Model file for the job. Use its own axes, mm. Round coordinates to 2 decimals unless told otherwise and drop trailing zeros. Loops run counter-clockwise (first coordinate to the right, second up) from the corner with the lowest first, then second, coordinate; pieces in that order, holes last. Notation, with made-up numbers: M 24.25,72 L 30.25,72 A8 ccw 30.25,82 Z; hole C 39.25,-1 d3. An arc over 180 degrees is marked long. Use a Markdown table: item, result. Add a question column.
Q1. Probe line 1 (X direction, y = -2, z = 36.5); line 2 (X direction, y = -4, z = 285). List the from-to ranges inside material, lowest first. Write a range as from..to.
Q2. Cut at B-B (x = 269.5). Give the cut face in (y, z), plus the area to 3 significant figures.
Q3. Cut at D-D (z = -49.5). Give the cut face in (x, y), plus the area to 3 significant figures.
Q4. Cut at A-A (z = 275). Give the cut face in (x, y).
Q5. Cut at C-C (y = -2.75). Give the cut face in (x, z), plus the area to 3 significant figures.
Q6. Pin check, flat tips, straight feed: pin 1 (1 mm diameter, centred on x = -131, y = -2, fed in from +Z); pin 2 (3 mm diameter, centred on x = 133.5, y = -1, fed in from -Z); pin 3 (1.5 mm diameter, centred on y = -2, z = 50.5, fed in from +X). Stop position of each tip, or through.
from build123d import *

# Parameters (mm, degrees)
BOSS_EXTRUDE1_DEPTH     = 6.35
CUT_EXTRUDE1_REACH      = 540.853
SKETCH3_R               = 48.260000044
MIRROR2_COPY_1_REACH    = 540.853
MIRROR2_COPY_1_SKETCH_R = 48.260000044
BOSS_EXTRUDE3_DEPTH     = 6.35
CUT_EXTRUDE12_DEPTH     = 55.372


with BuildPart() as part:
    # Sketch1 → Boss-Extrude1 (new body)
    with BuildSketch(Plane(origin=(0, 0, 0), x_dir=(1, 0, 0), z_dir=(0, 1, 0))):
        Polygon((254, -381), (-254, -381), (-381, -254), (-381, 254), (-254, 381), (254, 381), (381, 254), (381, -254), align=None)
    extrude(amount=-BOSS_EXTRUDE1_DEPTH)

    # Sketch3 → Cut-Extrude1 (cut, up to next)
    with BuildSketch(Plane(origin=(0, 0, 0), x_dir=(1, 0, 0), z_dir=(0, 1, 0)), mode=Mode.PRIVATE) as cut_extrude1_sk1:
        with BuildLine():
            Line((-175.260000044, -256.082305134), (-251.046104704, -331.868409794))
            Line((-251.046104704, -331.868409794), (-331.868409794, -251.046104704))
            Line((-331.868409794, -251.046104704), (-256.082305134, -175.260000044))
            Line((-256.082305134, -175.260000044), (-256.082305134, 0))
            Line((-256.082305134, 0), (-381, 0))
            Line((-381, 0), (-381, -254))
            Line((-381, -254), (-254, -381))
            Line((-254, -381), (0, -381))
            Line((0, -381), (0, -256.082305134))
            Line((0, -256.082305134), (-66.039999956, -256.082305134))
            Line((-66.039999956, -256.082305134), (-66.039999956, -279.4))
            ThreePointArc((-66.039999956, -279.4), (-120.65, -334.010000044), (-175.260000044, -279.4))
            Line((-175.260000044, -279.4), (-175.260000044, -256.082305134))
        make_face()
    cut_extrude1_tool1 = extrude(cut_extrude1_sk1.sketch, amount=-CUT_EXTRUDE1_REACH, mode=Mode.PRIVATE) & part.part
    # Sketch3 → Cut-Extrude1 (cut, up to next)
    with BuildSketch(Plane(origin=(0, 0, 0), x_dir=(1, 0, 0), z_dir=(0, 1, 0)), mode=Mode.PRIVATE) as cut_extrude1_sk2:
        with Locations(Location((-120.65, -279.4, 0), (0, 0, 270))):
            Circle(SKETCH3_R)
    cut_extrude1_tool2 = extrude(cut_extrude1_sk2.sketch, amount=-CUT_EXTRUDE1_REACH, mode=Mode.PRIVATE) & part.part
    cut_extrude1_1 = cut_extrude1_tool1.solids().sort_by_distance((-180.648154, 0, 267.741153))[0]
    add(cut_extrude1_1, mode=Mode.SUBTRACT)
    cut_extrude1_2 = cut_extrude1_tool2.solids().sort_by_distance((-120.65, 0, 279.4))[0]
    add(cut_extrude1_2, mode=Mode.SUBTRACT)
    cut_extrude1 = cut_extrude1_1 + cut_extrude1_2  # Cut-Extrude1 as one shape, for the pattern or mirror that repeats it

    # Mirror1: Cut-Extrude1 across plane
    add(cut_extrude1.mirror(Plane(origin=(0, 0, 0), x_dir=(0, 0, 1), z_dir=(1, 0, 0))), mode=Mode.SUBTRACT)

    # Mirror2: Cut-Extrude1 across plane
    add(cut_extrude1.mirror(Plane.XY), mode=Mode.SUBTRACT)

    # Mirror2 copy 1 sketch → Mirror2 copy 1 (cut, up to next)
    with BuildSketch(Plane(origin=(0, 0, 0), x_dir=(-1, 0, 0), z_dir=(0, 1, 0)), mode=Mode.PRIVATE) as mirror2_copy_1_sk1:
        with BuildLine():
            Line((-175.260000044, -256.082305134), (-251.046104704, -331.868409794))
            Line((-251.046104704, -331.868409794), (-331.868409794, -251.046104704))
            Line((-331.868409794, -251.046104704), (-256.082305134, -175.260000044))
            Line((-256.082305134, -175.260000044), (-256.082305134, 0))
            Line((-256.082305134, 0), (-381, 0))
            Line((-381, 0), (-381, -254))
            Line((-381, -254), (-254, -381))
            Line((-254, -381), (0, -381))
            Line((0, -381), (0, -256.082305134))
            Line((0, -256.082305134), (-66.039999956, -256.082305134))
            Line((-66.039999956, -256.082305134), (-66.039999956, -279.4))
            ThreePointArc((-66.039999956, -279.4), (-120.65, -334.010000044), (-175.260000044, -279.4))
            Line((-175.260000044, -279.4), (-175.260000044, -256.082305134))
        make_face()
    mirror2_copy_1_tool1 = extrude(mirror2_copy_1_sk1.sketch, amount=-MIRROR2_COPY_1_REACH, mode=Mode.PRIVATE) & part.part
    # Mirror2 copy 1 sketch → Mirror2 copy 1 (cut, up to next)
    with BuildSketch(Plane(origin=(0, 0, 0), x_dir=(-1, 0, 0), z_dir=(0, 1, 0)), mode=Mode.PRIVATE) as mirror2_copy_1_sk2:
        with Locations(Location((-120.65, -279.4, 0), (0, 0, 270))):
            Circle(MIRROR2_COPY_1_SKETCH_R)
    mirror2_copy_1_tool2 = extrude(mirror2_copy_1_sk2.sketch, amount=-MIRROR2_COPY_1_REACH, mode=Mode.PRIVATE) & part.part
    add(mirror2_copy_1_tool1.solids().sort_by_distance((180.648154, 0, -267.741153))[0], mode=Mode.SUBTRACT)
    add(mirror2_copy_1_tool2.solids().sort_by_distance((120.65, 0, -279.4))[0], mode=Mode.SUBTRACT)

    # Sketch39 → Boss-Extrude3 (add)
    with BuildSketch(Plane.XZ.offset(6.35)):
        with BuildLine():
            ThreePointArc((162.902960966, -256.082305134), (120.65, -231.139999956), (78.397039034, -256.082305134))
            Line((78.397039034, -256.082305134), (162.902960966, -256.082305134))
        make_face()
        with BuildLine():
            Line((-162.902960966, -256.082305134), (-78.397039034, -256.082305134))
            ThreePointArc((-78.397039034, -256.082305134), (-120.65, -231.139999956), (-162.902960966, -256.082305134))
        make_face()
    boss_extrude3 = extrude(amount=-BOSS_EXTRUDE3_DEPTH)

    # Sketch39_3 → Cut-Extrude12 (cut)
    with BuildSketch(Plane.XZ.offset(6.35)):
        with BuildLine():
            Line((78.397039034, -256.082305134), (66.039999956, -256.082305134))
            Line((66.039999956, -256.082305134), (66.039999956, -279.4))
            ThreePointArc((66.039999956, -279.4), (120.65, -334.010000044), (175.260000044, -279.4))
            Line((175.260000044, -279.4), (175.260000044, -256.082305134))
            Line((175.260000044, -256.082305134), (162.902960966, -256.082305134))
            ThreePointArc((162.902960966, -256.082305134), (167.384117635, -267.360487838), (168.910000044, -279.4))
            ThreePointArc((168.910000044, -279.4), (108.610487838, -326.134117635), (78.397039034, -256.082305134))
        make_face()
        with BuildLine():
            Line((-66.039999956, -279.4), (-66.039999956, -256.082305134))
            Line((-66.039999956, -256.082305134), (-78.397039034, -256.082305134))
            ThreePointArc((-78.397039034, -256.082305134), (-73.915882365, -267.360487838), (-72.389999956, -279.4))
            ThreePointArc((-72.389999956, -279.4), (-132.689512162, -326.134117635), (-162.902960966, -256.082305134))
            Line((-162.902960966, -256.082305134), (-175.260000044, -256.082305134))
            Line((-175.260000044, -256.082305134), (-175.260000044, -279.4))
            ThreePointArc((-175.260000044, -279.4), (-120.65, -334.010000044), (-66.039999956, -279.4))
        make_face()
    cut_extrude12 = extrude(amount=-CUT_EXTRUDE12_DEPTH, mode=Mode.SUBTRACT)

    # Mirror9: Boss-Extrude3, Cut-Extrude12 across plane
    add(boss_extrude3.mirror(Plane.XY))
    add(cut_extrude12.mirror(Plane.XY), mode=Mode.SUBTRACT)


solid = part.part
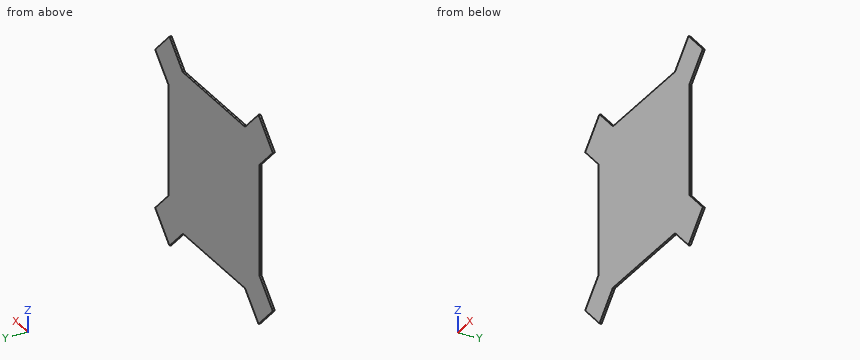
Checked values:
| question | item | result |
|---|---|---|
| 1 | line 1 | x = -256.08..256.08 |
| 1 | line 2 | x = -297.91..-204.18, 204.18..297.91 |
| 2 | outline | M -6.35,-313.41 L 0,-313.41 L 0,-188.68 L -6.35,-188.68 Z; M -6.35,188.68 L 0,188.68 L 0,313.41 L -6.35,313.41 Z |
| 2 | area | 1,580 mm^2 |
| 3 | outline | M -256.08,-6.35 L 256.08,-6.35 L 256.08,0 L -256.08,0 Z |
| 3 | area | 3,250 mm^2 |
| 4 | outline | M -307.91,-6.35 L -194.18,-6.35 L -194.18,0 L -307.91,0 Z; M 194.18,-6.35 L 307.91,-6.35 L 307.91,0 L 194.18,0 Z |
| 5 | outline | M -331.87,-251.05 L -251.05,-331.87 L -175.26,-256.08 L 175.26,-256.08 L 251.05,-331.87 L 331.87,-251.05 L 256.08,-175.26 L 256.08,175.26 L 331.87,251.05 L 251.05,331.87 L 175.26,256.08 L -175.26,256.08 L -251.05,331.87 L -331.87,251.05 L -256.08,175.26 L -256.08,-175.26 Z |
| 5 | area | 298,000 mm^2 |
| 6 | pin 1 | stops at z = 256.08 |
| 6 | pin 2 | stops at z = -256.08 |
| 6 | pin 3 | stops at x = 256.08 |
